Build history of the part. All positions in model axes, mm. A direction names the side the tool comes from. Round coordinates to 2 decimals unless told otherwise and drop trailing zeros. Order: outer loops, then holes, each group sorted by start corner. A loop starts at its lowest first (then second) coordinate and runs counter-clockwise, first axis right, second up. Notation, with made-up numbers: M 69.25,12 L 97.25,12 A31 ccw 97.25,40 Z; hole C 83.25,-9 d5. An arc over 180 degrees is marked long. One line per item, written item: value. Start each with the question number.
Item 1: Two-plate mould, pull along X, no slides. Class faces 3 (the flat face through (5, 123, 0)), 4 (the flat face through (-4.5, 0, -0.1)), 5 (the flat face through (0, 123, 4)): +X half, -X half, draft (parallel to the pull), parting line (faces both ways), or undercut.
Item 2: Band-saw the part on C-C, the plane x = 0. Give the number of separate pieces and of enclosed holes in the cut face, then the cut area to 3 significant figures.
Item 3: Band-saw the part on B-B, the plane y = 189.5. Write the cut outline in (x, z), then the cut area to 3 significant figures.
Item 4: Tool access for faces 1 (the flat face through (4, 123, 0)), 2 (the flat face through (-5, 123, 0)): list every direction of +Z, -Z, +X, -X, +Y, -Y with a clear straight run to the whole face (end or side of a thin tool).
Item 5: Pin check, flat tip, straight feed: pin 1 (1.8 mm diameter, centred on x = 0, y = 25, fed in from +Z). Stop position of the tip, or through.
Item 6: Probe L1, parallel to Y at x = 0, z = 4.55; L2, parallel to Z at x = 1.5, y = 185; L3, parallel to X at y = 225, z = 4.7. List the from-to ranges inside material, lowest first.
Item 7: Band-saw the part on A-A, the plane z = 0.5. Write the cut outline in (x, y).
```python
from build123d import *

# Parameters (mm, degrees)
SKETCH_1_W            = 10
SKETCH_1_H            = 10
SKETCH_1_W_2          = 8
SKETCH_1_H_2          = 8
EXTRUDE_1_DEPTH       = 250
HOLE_WIZARD_3_0_3_1_D = 3


with BuildPart() as part:
    # 草图1 → 凸台-拉伸1 (new body)
    with BuildSketch(Plane(origin=(0, 0, 0), x_dir=(1, 0, 0), z_dir=(0, 1, 0))):
        Rectangle(SKETCH_1_W, SKETCH_1_H)
        Rectangle(SKETCH_1_W_2, SKETCH_1_H_2, mode=Mode.SUBTRACT)
    extrude(amount=EXTRUDE_1_DEPTH)

    # Ø3.0 (3) 直径孔1 (through all)
    with Locations(Plane.XY.offset(5)):
        with Locations((0, 15), (0, 25)):
            hole_wizard_3_0_3_1 = Hole(HOLE_WIZARD_3_0_3_1_D / 2)

    # 镜向1: Ø3.0 (3) 直径孔1 across plane
    add(hole_wizard_3_0_3_1.mirror(Plane(origin=(0, 125, 0), x_dir=(0, 0, 1), z_dir=(0, -1, 0))), mode=Mode.SUBTRACT)


solid = part.part
```
Output:
1. face 3: +X half
1. face 4: draft
1. face 5: undercut
2. separate pieces: 10
2. enclosed holes: 0
2. area: 476 mm²
3. outline: M -5,-5 L 5,-5 L 5,5 L -5,5 Z; hole M -4,-4 L 4,-4 L 4,4 L -4,4 Z
3. area: 36.0 mm²
4. face 1: +Y, -Y
4. face 2: +Z, -Z, -X, +Y, -Y
5. pin 1: passes through
6. L1: y = 0 to 13.5, 16.5 to 23.5, 26.5 to 223.5, 226.5 to 233.5, 236.5 to 250
6. L2: z = -5 to -4, 4 to 5
6. L3: x = -5 to -1.5, 1.5 to 5
7. outline: M -5,0 L -4,0 L -4,250 L -5,250 Z; M 4,0 L 5,0 L 5,250 L 4,250 Z
